Geometry: final body of the model. Coordinates: model frame, mm. A direction names the side the tool comes from. Give positions to 0.01 mm unless a question says otherwise; leave off trailing zeros. Order: outer loops, then holes, each group sorted by start corner. A loop starts at its lowest first (then second) coordinate and runs counter-clockwise, first axis right, second up. Notation, with made-up numbers: (-13, 4) - (33, 4) arc R10 ccw to (33, 23) - close; hole circle Ø5 at (41, 80.25). An arc over 180 degrees is marked (long way). Use one line per item in the form item = value.
Autodesk Inventor part; units mm, degrees
ref_plane "YZ Plane" through (0, 0, 0) normal (1, 0, 0) x (0, 1, 0)
ref_plane "XZ Plane" through (0, 0, 0) normal (0, 1, 0) x (-1, 0, 0)
ref_plane "XY Plane" through (0, 0, 0) normal (0, 0, 1) x (1, 0, 0)
sketch "Sketch1" plane through (0, 0, 0) normal (0, 1, 0) x (-1, 0, 0)
  line L0 (-25.4, 4.953) -> (25.4, 4.953)
  line L1 (25.4, 4.953) -> (25.4, -4.953)
  line L2 (25.4, -4.953) -> (-25.4, -4.953)
  line L3 (-25.4, -4.953) -> (-25.4, 4.953)
  line L4 (-25.4, 4.953) -> (25.4, -4.953) construction
  line L5 (25.4, 4.953) -> (-25.4, -4.953) construction
  point P0 (0, 0)
  dimension "d0" = 50.8
  dimension "d1" = 9.906
extrude "Extrusion1" add sketch "Sketch1" along normal blind 4.826
sketch "Sketch2" plane through (-25.4, 0, 4.953) normal (0, 0, 1) x (1, 0, 0)
  line L0 (19.05, 0) -> (19.05, 2.54)
  line L1 (19.05, 2.54) -> (31.75, 2.54)
  line L2 (31.75, 2.54) -> (31.75, 0)
  line L3 (25.4, 0) -> (19.05, 2.54) construction
  line L4 (25.4, 0) -> (31.75, 2.54) construction
  line L5 (19.05, 0) -> (31.75, 0)
  line L6 (50.8, 0) -> (0, 0)
  point P0 (25.4, 0)
extrude "Extrusion2" cut sketch "Sketch2" against normal blind 12.7
sketch "Sketch3" plane through (25.4, 0, 4.953) normal (1, 0, 0) x (0, 0, -1)
  arc A0 (1.1698, 4.826) -> (8.7362, 4.826) centre (4.953, 0) ccw
  line L0 (0, 4.826) -> (9.906, 4.826)
  line L1 (1.1698, 4.826) -> (8.7362, 4.826)
extrude "Extrusion3" add sketch "Sketch3" along normal blind 6.35
sketch "Sketch4" plane through (-25.4, 0, -4.953) normal (-1, 0, 0) x (0, 0, 1)
  point P0 (4.953, 0)
sketch "Sketch5" plane through (-25.4, 0, -4.953) normal (-1, 0, 0) x (0, 0, 1)
  arc A0 (4.1541, 4.8522) -> (5.7772, 4.826) centre (4.953, 4.0539) ccw
  line L0 (9.906, 1.595) -> (0, 1.595)
  line L1 (9.906, 0) -> (0, 0)
  line L2 (4.1541, 4.8522) -> (5.7772, 4.826)
  line L3 (1.1698, 4.826) -> (8.7362, 4.826)
  point P0 (4.953, 0)
revolve "Revolution1" add sketch "Sketch5" angle 90 about axis through (-25.4, 1.595, 4.953) along (0, 0, 1)
properties part number "pig_nose_tail"
(1) Cut plane A-A on z = -2. Output: boundary loops of the cut face in (x, y), plus the area to 3 significant figures.
Computed values:
outline = (-25.4, 0) - (-6.35, 0) - (-6.35, 2.54) - (6.35, 2.54) - (6.35, 0) - (25.4, 0) - (25.4, -5.8) - (31.75, -5.8) - (31.75, 4.83) - (-25.4, 4.83) - close
area = 280 mm²
(2) Cut plane C-C on y = -3.25. Output: boundary loops of the cut face in (x, z), plus the area to 3 significant figures.
Computed values:
outline = (25.4, -5.2) - (31.75, -5.2) - (31.75, 5.2) - (25.4, 5.2) - close
area = 66.0 mm²
(3) Ray query, line 1 along X through (y, z) = (2.5, -2.25); line 2 along Y through (x, z) = (10.5, -2.75); line 3 along Z through (x, y) = (-7.5, 4). Return the intervals inside material, ascending.
Computed values:
line_1 = -25.4 to -6.35, 6.35 to 31.75
line_2 = 0 to 4.83
line_3 = -4.95 to 4.95
(4) Contact query for flat-ended pins moving along their axis: pin 1 Ø3 at (y, z) = (0, -1) entering from -X; pin 2 Ø5 at (x, z) = (14.5, 4) entering from -Y; pin 3 Ø1.5 at (x, y) = (25, -2) entering from +Z. Output: stop coordinate, or through.
Computed values:
pin_1 = -25.4
pin_2 = 0
pin_3 = 5.98
(5) Reachability of faces 1 (the face through (25.4, 4.5, 4.6)), 2 (the face through (0, 2.54, 0)), 3 (the face through (25.4, 4.5, -4.6)) from +Z, -Z, +X, -X, +Y, -Y: full face, straight path, thin tool, end or side. Return the list, or none.
Computed values:
face_1 = +Z, +X, +Y
face_2 = +Z, -Z, -Y
face_3 = -Z, +X, +Y
(6) Cut plane B-B on x = -13. Output: boundary loops of the cut face in (y, z).
Computed values:
outline = (0, -4.95) - (4.83, -4.95) - (4.83, 4.95) - (0, 4.95) - close
(7) Pull-direction query (X, two-part tool) for faces 4 (the face through (-27.72, 3.86, 0)), 5 (the face through (0, 3, -4.953)), 6 (the face through (6.35, 1, 0)); classes: released by +X, released by -X, zero draft, split by the parting line, or undercut.
Computed values:
face_4 = released by -X
face_5 = zero draft
face_6 = undercut
(8) Cut plane D-D on z = 2.5. Output: boundary loops of the cut face in (x, y), plus the area to 3 significant figures.
Computed values:
outline = (-25.4, 0) - (-6.35, 0) - (-6.35, 2.54) - (6.35, 2.54) - (6.35, 0) - (25.4, 0) - (25.4, -5.6) - (31.75, -5.6) - (31.75, 4.83) - (-25.4, 4.83) - close
area = 279 mm²
